Part model, mm, in its own coordinate system. A direction names the side the tool comes from. Give positions to 0.01 mm unless a question says otherwise; leave off trailing zeros. Write each loop counter-clockwise with the first axis right and the second up, starting at its lowest first coordinate (ties: lowest second). Pieces come first, ordered by that corner, then holes. Notation, with made-up numbers: M 66,71.25 L 91,71.25 A24 cw 91,102.25 Z; hole C 8,82 d9. An arc over 180 degrees is marked long. Use CSV: the item, a comma, the result in double quotes. Start each with the question number.
Item 1: Cut at B-B (x = -1). List the corners of the cut face in (y, z), then the cut area to 3 significant figures.
Item 2: Pin check, flat tips, straight feed: pin 1 (5 mm diameter, centred on y = 19.5, z = 4.5, fed in from +X); pin 2 (2 mm diameter, centred on y = 26, z = -4.5, fed in from +X); pin 3 (3 mm diameter, centred on y = 33, z = 2.5, fed in from -X) (3 decimals). Stop position of each tip, or through.
Item 3: Which spindle directions (+Z, -Z, +X, -X, +Y, -Y) get a long thin tool onto all of the face, cutting with end or side? Do faces 1 (the flat face through (5.48, 33.52, 3.21)), 2 (the flat face through (0, 34, 3.6)). Say none if no direction does.
Item 4: Cut at A-A (y = 25). List the corners of the cut face in (x, z).
Item 5: Mould opens along Z. For faces 3 (the flat face through (3, 34, 2)), 4 (the flat face through (3, 0, 3)), 5 (the flat face through (-5.48, 33.52, -3.21)) say: released by +Z, released by -Z, zero draft, split by the parting line, or undercut.
Item 6: Cut at C-C (z = 5.25). List the corners of the cut face in (x, y), then the cut area to 3 significant figures.
Item 7: Drill centre lines: line 1 (Z direction, x = 2, y = 48); line 2 (Z direction, x = -1.5, y = 27); line 3 (Z direction, x = 2.5, y = 18). Where is each one in solid material? Low to high. Write a range as [from, to].
from build123d import *

# Parameters (mm, degrees)
BOSS_EXTRUDE1_DEPTH = 68
SKETCH2_R           = 0.5
CUT_EXTRUDE1_DEPTH  = 69.68832385
FILLET1_R           = 1


with BuildPart() as part:
    # Sketch1 → Boss-Extrude1 (new body)
    with BuildSketch(Plane(origin=(0, 0, 0), x_dir=(1, 0, 0), z_dir=(0, 1, 0))):
        Polygon((3.666174209, 6.35), (-3.666174209, 6.35), (-7.332348419, 0), (-3.666174209, -6.35), (3.666174209, -6.35), (7.332348419, 0), align=None)
        Polygon((2.078460969, 3.6), (-2.078460969, 3.6), (-4.156921938, 0), (-2.078460969, -3.6), (2.078460969, -3.6), (4.156921938, 0), align=None, mode=Mode.SUBTRACT)
    extrude(amount=BOSS_EXTRUDE1_DEPTH)

    # Sketch2 → Cut-Extrude1 (cut, through all)
    with BuildSketch(Plane(origin=(0, 68, 0), x_dir=(1, 0, 0), z_dir=(0, 1, 0))):
        with Locations((-2.078460969, 3.6)):
            Circle(SKETCH2_R)
        with Locations((2.078460969, 3.6)):
            Circle(SKETCH2_R)
        with Locations((4.156921938, 0)):
            Circle(SKETCH2_R)
        with Locations((2.078460969, -3.6)):
            Circle(SKETCH2_R)
        with Locations((-2.078460969, -3.6)):
            Circle(SKETCH2_R)
        with Locations((-4.156921938, 0)):
            Circle(SKETCH2_R)
    extrude(amount=-CUT_EXTRUDE1_DEPTH, mode=Mode.SUBTRACT)

    # Fillet1
    fillet1_edges = [part.edges().sort_by_distance(p)[0] for p in [
        (7.332348419, 34, 0),
        (3.666174209, 34, 6.35),
        (-3.666174209, 34, 6.35),
        (-7.332348419, 34, 0),
        (-3.666174209, 34, -6.35),
        (3.666174209, 34, -6.35),
    ]]
    fillet(fillet1_edges, radius=FILLET1_R)


solid = part.part
Worked answers:
1,outline,"M 0,-6.35 L 68,-6.35 L 68,-3.6 L 0,-3.6 Z; M 0,3.6 L 68,3.6 L 68,6.35 L 0,6.35 Z"
1,area,"374 mm^2"
2,pin 1,"stops at x = 6.18"
2,pin 2,"stops at x = 5.31"
2,pin 3,"stops at x = -6.755"
3,face 1,"+Z, +X, +Y, -Y"
3,face 2,"+Y, -Y"
4,outline,"M -7.04,-0.5 L -3.95,-5.85 A1 ccw -3.09,-6.35 L 3.09,-6.35 A1 ccw 3.95,-5.85 L 7.04,-0.5 A1 ccw 7.04,0.5 L 3.95,5.85 A1 ccw 3.09,6.35 L -3.09,6.35 A1 ccw -3.95,5.85 L -7.04,0.5 A1 ccw Z; hole M -3.91,-0.43 L -2.33,-3.17 A0.5 ccw long -1.58,-3.6 L 1.58,-3.6 A0.5 ccw long 2.33,-3.17 L 3.91,-0.43 A0.5 ccw long 3.91,0.43 L 2.33,3.17 A0.5 ccw long 1.58,3.6 L -1.58,3.6 A0.5 ccw long -2.33,3.17 L -3.91,0.43 A0.5 ccw long Z"
5,face 3,"undercut"
5,face 4,"zero draft"
5,face 5,"released by -Z"
6,outline,"M -4.3,0 L 4.3,0 L 4.3,68 L -4.3,68 Z"
6,area,"585 mm^2"
7,line 1,"z = [-6.35, -4.09], [4.09, 6.35]"
7,line 2,"z = [-6.35, -3.6], [3.6, 6.35]"
7,line 3,"z = [-6.35, -3.87], [-3.33, -2.87], [2.87, 3.33], [3.87, 6.35]"
